CAD build for the part. Positions are in the model's coordinates, mm. Face numbers are marked on the shaded views. A direction names the side the tool comes from. Give positions to 0.01 mm unless a question says otherwise; leave off trailing zeros. Write each loop counter-clockwise with the first axis right and the second up, starting at its lowest first coordinate (ties: lowest second). Pieces come first, ordered by that corner, then holes. Notation, with made-up numbers: (58, 24.25) - (68, 24.25) arc R17 ccw to (68, 37.25) - close; hole circle Ø6 at (67, -14). An arc over 180 degrees is marked (long way). Put each result on its own line as item: value. Start each with the question number.
1. Tool access for the marked faces 5, 6 and 7: list every direction of +Z, -Z, +X, -X, +Y, -Y with a clear straight run to the whole face (end or side of a thin tool).
2. Cut at B-B on x = 0. List the corners of the cut face in (y, z), and give its area (3 significant figures).
3. Cut at C-C on y = -15.5. List the corners of the cut face in (x, z), and give its area (3 significant figures).
4. Cut at A-A on z = 12.5. List the corners of the cut face in (x, y), and give its area (3 significant figures).
5. Wall check: line 1 (Y direction, x = 0, z = 6.75); line 2 (Z direction, x = -14, y = -9); line 3 (Y direction, x = 0, z = 1.4). Give the ranges that are in metal, low to high.
6. Cut at D-D on x = -18.5. List the corners of the cut face in (y, z).
7. Drop flat-ended pins along their axis: pin 1 (5 mm diameter, centred on x = -16, z = 10, fed in from -Y); pin 2 (8 mm diameter, centred on x = 26, y = -7, fed in from +Z); pin 3 (8 mm diameter, centred on x = 6.5, y = 6, fed in from -Z); pin 4 (10 mm diameter, centred on x = -16.51, y = 0, fed in from +Z). Give the stop position or say it passes through.
8. Mould opens along Y. For the marked faces 1, 2, 3 and 4 say: +Y half, -Y half, draft (parallel to the pull), parting line (faces both ways), or undercut.
from build123d import *

# Parameters (mm, degrees)
F0_R     = 38.1
F1_DEPTH = 15.24
F2_R     = 31.75
F3_DEPTH = 3.81
F4_R     = 31.75
F5_DEPTH = 3.81
F6_R     = 6.35
F7_DEPTH = 11.431
F8_W     = 2.54
F8_H     = 12.7


# Not quite as in the source:
# - a feature names something its author has since deleted; it is built from what else it names


with BuildPart() as f1:
    # F0 (on Top) → F1 (new body)
    with BuildSketch(Plane.XY):
        Circle(F0_R)
    extrude(amount=F1_DEPTH)

    # F2 (on face) → F3 (cut)
    with BuildSketch(Plane.XY.offset(15.24)):
        Circle(F2_R)
    extrude(amount=-F3_DEPTH, mode=Mode.SUBTRACT)

    # F4 (on face) → F5 (cut)
    with BuildSketch(Plane(origin=(0, 0, 0), x_dir=(1, 0, 0), z_dir=(0, 0, -1))):
        Circle(F4_R)
    extrude(amount=-F5_DEPTH, mode=Mode.SUBTRACT)

    # F6 (on face) → F7 (cut, through all)
    with BuildSketch(Plane.XY.offset(11.43)):
        with Locations((0, 16.51)):
            Circle(F6_R)
        with Locations((16.51, 0)):
            Circle(F6_R)
        with Locations((0, -16.51)):
            Circle(F6_R)
        with Locations((-16.51, 0)):
            Circle(F6_R)
    extrude(amount=-F7_DEPTH, mode=Mode.SUBTRACT)

    # F8 (on Front) → F10 (revolve)
    with BuildSketch(Plane.XZ):
        with Locations((1.27, 17.78)):
            Rectangle(F8_W, F8_H)
    revolve(axis=Axis((0, 0, 19.05), (0, 0, -1)))


solid = f1.part
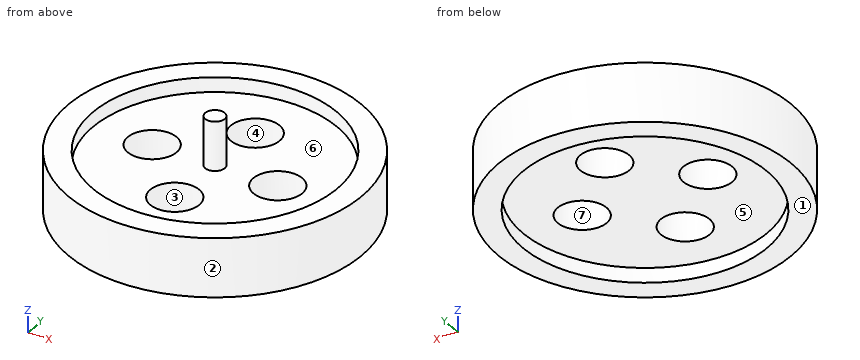
Report:
1. face 5: -Z
1. face 6: +Z
1. face 7: +Z, -Z
2. outline: (-38.1, 0) - (-31.75, 0) - (-31.75, 3.81) - (-22.86, 3.81) - (-22.86, 11.43) - (-31.75, 11.43) - (-31.75, 15.24) - (-38.1, 15.24) - close; (-10.16, 3.81) - (10.16, 3.81) - (10.16, 11.43) - (2.54, 11.43) - (2.54, 24.13) - (-2.54, 24.13) - (-2.54, 11.43) - (-10.16, 11.43) - close; (22.86, 3.81) - (31.75, 3.81) - (31.75, 0) - (38.1, 0) - (38.1, 15.24) - (31.75, 15.24) - (31.75, 11.43) - (22.86, 11.43) - close
2. area: 548 mm²
3. outline: (-34.8, 0) - (-27.71, 0) - (-27.71, 3.81) - (-6.27, 3.81) - (-6.27, 11.43) - (-27.71, 11.43) - (-27.71, 15.24) - (-34.8, 15.24) - close; (6.27, 3.81) - (27.71, 3.81) - (27.71, 0) - (34.8, 0) - (34.8, 15.24) - (27.71, 15.24) - (27.71, 11.43) - (6.27, 11.43) - close
3. area: 543 mm²
4. outline: circle Ø76.2 at (0, 0); circle Ø5.08 at (0, 0); hole circle Ø63.5 at (0, 0)
4. area: 1,410 mm²
5. line 1: y = -38.1 to -22.86, -10.16 to 10.16, 22.86 to 38.1
5. line 2: z = 3.81 to 11.43
5. line 3: y = -38.1 to -31.75, 31.75 to 38.1
6. outline: (-33.31, 0) - (-25.8, 0) - (-25.8, 3.81) - (-6.03, 3.81) - (-6.03, 11.43) - (-25.8, 11.43) - (-25.8, 15.24) - (-33.31, 15.24) - close; (6.03, 3.81) - (25.8, 3.81) - (25.8, 0) - (33.31, 0) - (33.31, 15.24) - (25.8, 15.24) - (25.8, 11.43) - (6.03, 11.43) - close
7. pin 1: stops at y = -35.63
7. pin 2: stops at z = 11.43
7. pin 3: stops at z = 3.81
7. pin 4: passes through
8. face 1: draft
8. face 2: parting line
8. face 3: undercut
8. face 4: undercut
